from build123d import *

# Parameters (mm, degrees)
BOSS_EXTRUDE2_DEPTH = 23


with BuildPart() as part:
    # Sketch1 → Revolve-Thin3 (revolve)
    with BuildSketch(Plane.XY, mode=Mode.PRIVATE) as revolve_thin3_sk:
        Polygon((-20, 13.228756555), (-18, 13.228756555), (-9, 0), (-9, -10), (-11, -10), (-11, -0.615831877), (-19.058300524, 11.228756555), (-20, 11.228756555), align=None)
    revolve(revolve_thin3_sk.sketch.rotate(Axis((0, 0, 0), (0, 1, 0)), 270), axis=Axis((0, 0, 0), (0, 1, 0)))



with BuildPart() as body_2:
    # Sketch7 → Revolve2 (revolve)
    with BuildSketch(Plane.XY, mode=Mode.PRIVATE) as revolve2_sk:
        Polygon((0, 18.228756555), (18, 36.228756555), (20, 36.228756555), (20, 39.05718368), (18, 39.05718368), (0, 21.05718368), align=None)
    revolve(revolve2_sk.sketch.rotate(Axis((0, 0, 0), (0, 1, 0)), 270), axis=Axis((0, 0, 0), (0, 1, 0)))


with BuildPart() as part_1:
    add(part.part)

    add(body_2.part)  # Boss-Extrude2 merges body 2
    # Sketch8 → Boss-Extrude2 (add)
    with BuildSketch(Plane.XZ.offset(-36.228756555)):
        Polygon((-16.024377741, -8.198738805), (-16.898983319, -6.198738805), (-18.776648132, -6.887487561), (-16.684330841, -11.028739927), (-15.015897757, -9.925865935), align=None)
        Polygon((16.015573595, 8.215923712), (15.005241471, 9.941968034), (16.672490524, 11.046631149), (18.697980652, 7.098275814), (16.828182587, 6.388448233), align=None)
    extrude(amount=BOSS_EXTRUDE2_DEPTH)


solid = part_1.part
Read the model definition and answer for the solid it produces. Units are mm, in the model's axes. A direction names the side the tool comes from. Coordinates: 2 decimals unless noted, no trailing zeros. Write each loop counter-clockwise with the first axis right and the second up, starting at its lowest first coordinate (ties: lowest second). Pieces come first, ordered by that corner, then holes. Notation, with made-up numbers: (-20.5, -24.75) -> (9.5, -24.75) arc R22 ccw to (9.5, -15.75) -> close; hole circle Ø4 at (-33.75, 89.25). An arc over 180 degrees is marked (long way). Return JSON: item names as keys, results as strings.
(1) The part is cut by section B-B on y = -4. Give the vertices of the cut face in (x, z), then the cut area to 3 significant figures.
Answers below:
{"outline": "circle Ø22 at (0, 0); hole circle Ø18 at (0, 0)", "area": "126 mm^2"}
(2) The part is cut by section D-D on y = 4.5. Give the vertices of the cut face in (x, z), then the cut area to 3 significant figures.
Answers below:
{"outline": "circle Ø28.96 at (0, 0); hole circle Ø24.12 at (0, 0)", "area": "202 mm^2"}
(3) Consider line 1 along X through (y, z) = (-6.25, 0); line 2 along X through (y, z) = (34, -7.5); line 3 along Y through (x, z) = (18, 6.5). Determine where each line is inside the solid, lowest interval first. Write a range as from..to.
Answers below:
{"line 1": "-11..-9, 9..11", "line 2": "-18.47..-16.33, -13.87..-10.55, 10.55..13.87", "line 3": "11.23..13.23, 36.23..39.06"}
(4) The part is cut by section C-C on x = 7.5. State how many separate pieces and enclosed holes the cut face has, then the cut area to 3 significant figures.
Answers below:
{"separate pieces": "3", "enclosed holes": "0", "area": "245 mm^2"}
(5) Each of these flat-tipped pins is pushed along its axis until it touches: P1, Ø0.6, axis at x = -17.5, z = -8, coming from the -Y side; P2, Ø12, axis at y = 29.5, z = 12.5, coming from the -X side; P3, Ø2, axis at x = 18, z = 8.5, coming from the -Y side. Where does it stop, or does it pass through?
Answers below:
{"P1": "y = 11.06", "P2": "x = -13.45", "P3": "y = 11"}
(6) Which of the six approach directions +Z, -Z, +X, -X, +Y, -Y give full straight-line access (tool end or side, diameter ignored) to faces 1 (the flat face through (9, -10, 2)), 2 (the flat face through (15.83, 24.89, 10.49)), 3 (the cylindrical face through (-2.703, -5.07, -8.584)), 4 (the flat face through (17.67, 24.89, 9.1))?
Answers below:
{"face 1": "+Z, -Z, +X, -X, -Y", "face 2": "+Z", "face 3": "-Y", "face 4": "+Z, +X"}
(7) The part is cut by section A-A on y = 31. Give the vertices of the cut face in (x, z).
Answers below:
{"outline": "(-18.78, -6.89) -> (-16.68, -11.03) -> (-15.02, -9.93) -> (-16.02, -8.2) -> (-16.9, -6.2) -> close; circle Ø25.54 at (0, 0); (15.01, 9.94) -> (16.02, 8.22) -> (16.83, 6.39) -> (18.7, 7.1) -> (16.67, 11.05) -> close; hole circle Ø19.89 at (0, 0)"}
(8) For a pull along X with two mould halves and no side action, classify faces 5 (the flat face through (-15.862, 24.89, -10.485)), 6 (the flat face through (-17.825, 24.89, -6.538)), 7 (the flat face through (-7, 13.229, 17)) as pulls with the +X half, pulls with the -X half, needs draft (parallel to the pull), parting line crosses it, or undercut.
Answers below:
{"face 5": "undercut", "face 6": "pulls with the -X half", "face 7": "needs draft"}
